Source: CAD feature listing. Evaluate the final solid. Frame: model axes, mm. Give positions to 0.01 mm unless a question says otherwise; leave off trailing zeros. Write each loop counter-clockwise with the first axis right and the second up, starting at its lowest first coordinate (ties: lowest second). Pieces come first, ordered by that corner, then holes. Notation, with made-up numbers: (67, -32) -> (81, -32) arc R17 cw to (81, -7) -> close; hole circle Ø10 at (4.25, 12). An arc over 180 degrees is marked (long way). Write item = value, one per line.
from build123d import *

# Parameters (mm, degrees)
BOSS_EXTRUDE2_DEPTH     = 6.35
CUT_EXTRUDE1_REACH      = 132.909
CUT_EXTRUDE2_DEPTH      = 131.908603613
CUT_EXTRUDE2_DEPTH_BACK = 131.908603613
SKETCH5_R               = 3.175


with BuildPart() as part:
    # Sketch3 → Boss-Extrude2 (new body)
    with BuildSketch(Plane(origin=(0, 0, 0), x_dir=(0, 0, -1), z_dir=(1, 0, 0))):
        with BuildLine():
            Line((-57.15, -114.3), (57.15, -114.3))
            ThreePointArc((57.15, -114.3), (61.640128061, -112.440128061), (63.5, -107.95))
            Line((63.5, -107.95), (63.5, 107.95))
            ThreePointArc((63.5, 107.95), (61.640128061, 112.440128061), (57.15, 114.3))
            Line((57.15, 114.3), (-57.15, 114.3))
            ThreePointArc((-57.15, 114.3), (-61.640128061, 112.440128061), (-63.5, 107.95))
            Line((-63.5, 107.95), (-63.5, -107.95))
            ThreePointArc((-63.5, -107.95), (-61.640128061, -112.440128061), (-57.15, -114.3))
        make_face()
        with BuildLine():
            Line((-31.75, -76.2), (31.75, -76.2))
            ThreePointArc((31.75, -76.2), (36.240128061, -74.340128061), (38.1, -69.85))
            Line((38.1, -69.85), (38.1, 69.85))
            ThreePointArc((38.1, 69.85), (36.240128061, 74.340128061), (31.75, 76.2))
            Line((31.75, 76.2), (-31.75, 76.2))
            ThreePointArc((-31.75, 76.2), (-36.240128061, 74.340128061), (-38.1, 69.85))
            Line((-38.1, 69.85), (-38.1, -69.85))
            ThreePointArc((-38.1, -69.85), (-36.240128061, -74.340128061), (-31.75, -76.2))
        make_face(mode=Mode.SUBTRACT)
    extrude(amount=BOSS_EXTRUDE2_DEPTH)

    # Sketch4 → Cut-Extrude1 (cut, up to next)
    with BuildSketch(Plane(origin=(6.35, 0, 0), x_dir=(0, 0, -1), z_dir=(1, 0, 0)), mode=Mode.PRIVATE) as cut_extrude1_sk1:
        Polygon((0, -101.6), (-8.980256121, -92.619743879), (-9.878281733, -93.517769491), (0, -103.396051224), (9.878281733, -93.517769491), (8.980256121, -92.619743879), align=None)
    cut_extrude1_tool1 = extrude(cut_extrude1_sk1.sketch, amount=-CUT_EXTRUDE1_REACH, mode=Mode.PRIVATE) & part.part
    add(cut_extrude1_tool1.solids().sort_by_distance((6.35, -97.269002, 4.649259))[0], mode=Mode.SUBTRACT)

    # Sketch5 → Cut-Extrude2 (cut, two sides: drawn at the far end of the back side and taken through both)
    with BuildSketch(Plane(origin=(6.35, 0, 0), x_dir=(0, 0, -1), z_dir=(1, 0, 0)).offset(-CUT_EXTRUDE2_DEPTH_BACK)):
        with Locations((-31.75, 93.472)):
            Circle(SKETCH5_R)
        with Locations((31.75, 93.472)):
            Circle(SKETCH5_R)
    extrude(amount=CUT_EXTRUDE2_DEPTH + CUT_EXTRUDE2_DEPTH_BACK, mode=Mode.SUBTRACT)


solid = part.part
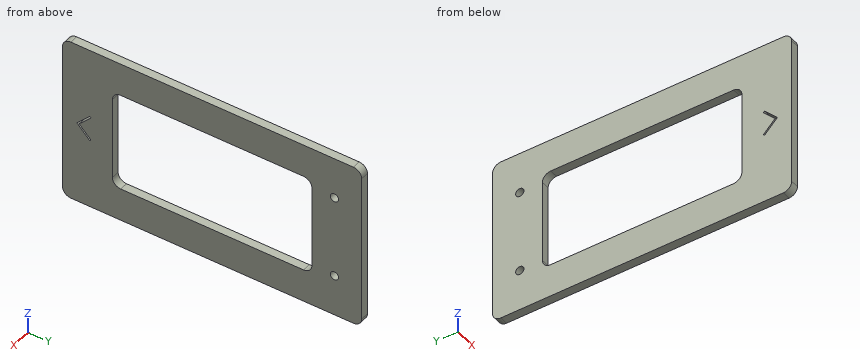
1) Cut plane B-B (x = 1). Return the cut outline in (y, z) (3 decimals), then the cut area to 3 significant figures.
Computed:
outline = (-114.3, -57.15) arc R6.35 ccw to (-107.95, -63.5) -> (107.95, -63.5) arc R6.35 ccw to (114.3, -57.15) -> (114.3, 57.15) arc R6.35 ccw to (107.95, 63.5) -> (-107.95, 63.5) arc R6.35 ccw to (-114.3, 57.15) -> close; hole (-103.396, 0) -> (-93.518, -9.878) -> (-92.62, -8.98) -> (-101.6, 0) -> (-92.62, 8.98) -> (-93.518, 9.878) -> close; hole (-76.2, -31.75) arc R6.35 ccw to (-69.85, -38.1) -> (69.85, -38.1) arc R6.35 ccw to (76.2, -31.75) -> (76.2, 31.75) arc R6.35 ccw to (69.85, 38.1) -> (-69.85, 38.1) arc R6.35 ccw to (-76.2, 31.75) -> close; hole circle Ø6.35 at (93.472, -31.75); hole circle Ø6.35 at (93.472, 31.75)
area = 17,300 mm²
2) Cut plane A-A (y = 40). Return the cut outline in (x, z).
Computed:
outline = (0, -63.5) -> (6.35, -63.5) -> (6.35, -38.1) -> (0, -38.1) -> close; (0, 38.1) -> (6.35, 38.1) -> (6.35, 63.5) -> (0, 63.5) -> close
3) Material intervals for L1, parallel to Y at x = 2, z = 31.75; L2, parallel to Z at x = 2.5, y = -37.5; L3, parallel to Y at x = 1.5, z = 7.5, sorted ascending.
Computed:
L1 = -114.3 to -76.2, 76.2 to 90.3, 96.65 to 114.3
L2 = -63.5 to -38.1, 38.1 to 63.5
L3 = -114.3 to -95.9, -94.1 to -76.2, 76.2 to 114.3
